Work out the finished part from the listing and answer in its coordinate system (mm). Coordinates: 2 decimals unless noted, no trailing zeros. Order: outer loops, then holes, each group sorted by start corner. A loop starts at its lowest first (then second) coordinate and runs counter-clockwise, first axis right, second up. Notation, with made-up numbers: M 66,20 L 93,20 A17 cw 93,24 Z; hole C 35,-15 d1. An arc over 180 degrees is marked long. Use a Markdown table: item, result.
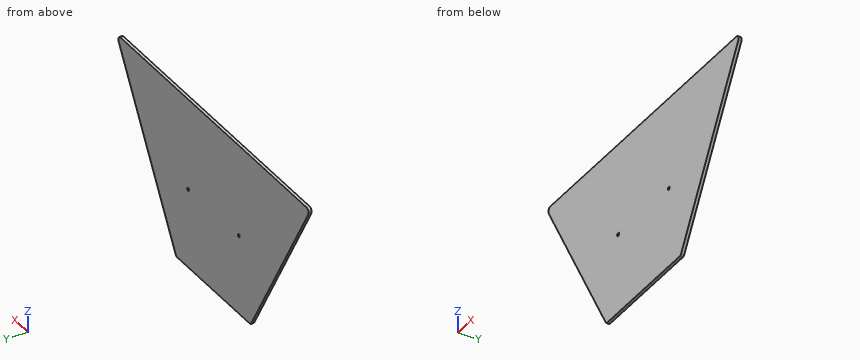
from build123d import *

# Parameters (mm, degrees)
BOSS_EXTRUDE1_DEPTH = 3.175
FILLET1_R           = 3.81
FILLET2_R           = 2.54
SKETCH2_R           = 1.651
CUT_EXTRUDE1_DEPTH  = 4.175


with BuildPart() as part:
    # Sketch1 → Boss-Extrude1 (new body)
    with BuildSketch(Plane(origin=(0, 0, 0), x_dir=(1, 0, 0), z_dir=(0, 1, 0))):
        Polygon((0, 0), (165.1, 0), (63.5, 177.8), (0, 177.8), align=None)
    boss_extrude1 = extrude(amount=BOSS_EXTRUDE1_DEPTH)

    # Mirror1: Boss-Extrude1 across plane
    add(boss_extrude1.mirror(Plane(origin=(0, 0, 0), x_dir=(0, 0, 1), z_dir=(1, 0, 0))))

    # Fillet1
    fillet1_edges = [part.edges().sort_by_distance(p)[0] for p in [
        (-165.1, 1.5875, 0),
        (165.1, 1.5875, 0),
    ]]
    fillet(fillet1_edges, radius=FILLET1_R)

    # Fillet2
    fillet2_edges = [part.edges().sort_by_distance(p)[0] for p in [
        (-63.5, 1.5875, -177.8),
        (63.5, 1.5875, -177.8),
    ]]
    fillet(fillet2_edges, radius=FILLET2_R)

    # Sketch2 → Cut-Extrude1 (cut, through all)
    with BuildSketch(Plane(origin=(0, 3.175, 0), x_dir=(1, 0, 0), z_dir=(0, 1, 0))):
        with Locations((43.18, 95.25)):
            Circle(SKETCH2_R)
    cut_extrude1 = extrude(amount=-CUT_EXTRUDE1_DEPTH, mode=Mode.SUBTRACT)

    # Mirror2: Cut-Extrude1 across plane
    add(cut_extrude1.mirror(Plane(origin=(0, 0, 0), x_dir=(0, 0, 1), z_dir=(1, 0, 0))), mode=Mode.SUBTRACT)


solid = part.part
(1) A cutting plane is placed at C-C (x = 86). Determine the outline of the cut face in (y, z) (3 decimals), then the cut area to 4 significant figures.
Conclusion:
| item | result |
|---|---|
| outline | M 0,-138.425 L 3.175,-138.425 L 3.175,0 L 0,0 Z |
| area | 439.5 mm2 |
(2) A cutting plane is placed at B-B (z = -156). Determine the outline of the cut face in (x, y) (3 decimals).
Conclusion:
| item | result |
|---|---|
| outline | M -75.957,0 L 75.957,0 L 75.957,3.175 L -75.957,3.175 Z |
(3) Straight lines are drawn through the part: L1, parallel to Z at x = 43.18, y = 2.4; L2, parallel to X at y = 1.9, z = -95.25; L3, parallel to X at y = 2.6, z = -60.5. For each, find the intervals that lie inside material, in ascending order.
Conclusion:
| item | result |
|---|---|
| L1 | -177.8 to -96.9, -93.6 to 0 |
| L2 | -110.67 to -44.83, -41.53 to 41.53, 44.83 to 110.67 |
| L3 | -130.53 to 130.53 |
(4) A cutting plane is placed at A-A (y = 0.95). Determine the outline of the cut face in (x, z), then the cut area to 3 significant figures.
Conclusion:
| item | result |
|---|---|
| outline | M -161.84,-5.7 L -64.23,-176.52 A2.54 ccw -62.03,-177.8 L 62.03,-177.8 A2.54 ccw 64.23,-176.52 L 161.84,-5.7 A3.81 ccw 158.53,0 L -158.53,0 A3.81 ccw Z; hole C -43.18,-95.25 d3.3; hole C 43.18,-95.25 d3.3 |
| area | 40,600 mm2 |
